```python
from build123d import *

# Parameters (mm, degrees)
SKETCH_1_W      = 45
SKETCH_1_H      = 16
SKETCH_1_R      = 0.5
EXTRUDE_1_DEPTH = 2
EXTRUDE_2_DEPTH = 20
SKETCH_3_W      = 45
SKETCH_3_H      = 16
SKETCH_3_R      = 0.5
EXTRUDE_3_DEPTH = 2


with BuildPart() as part:
    # 草图1 → 凸台-拉伸1 (new body)
    with BuildSketch(Plane.XY):
        Rectangle(SKETCH_1_W, SKETCH_1_H)
        with Locations((-20, -6.5)):
            Circle(SKETCH_1_R, mode=Mode.SUBTRACT)
        with Locations((-20, 6.5)):
            Circle(SKETCH_1_R, mode=Mode.SUBTRACT)
        with Locations((20, 6.5)):
            Circle(SKETCH_1_R, mode=Mode.SUBTRACT)
        with Locations((20, -6.5)):
            Circle(SKETCH_1_R, mode=Mode.SUBTRACT)
    extrude(amount=EXTRUDE_1_DEPTH)

    # 草图2 → 凸台-拉伸2 (add)
    with BuildSketch(Plane.XY.offset(2)):
        Polygon((-18.845299462, 6.5), (-19.422649731, 7.5), (-20.577350269, 7.5), (-21.154700538, 6.5), (-20.577350269, 5.5), (-19.422649731, 5.5), align=None)
        Polygon((19.422649731, 5.5), (18.845299462, 6.5), (19.422649731, 7.5), (20.577350269, 7.5), (21.154700538, 6.5), (20.577350269, 5.5), align=None)
        Polygon((18.845299462, -6.5), (19.422649731, -7.5), (20.577350269, -7.5), (21.154700538, -6.5), (20.577350269, -5.5), (19.422649731, -5.5), align=None)
        Polygon((-19.422649731, -5.5), (-18.845299462, -6.5), (-19.422649731, -7.5), (-20.577350269, -7.5), (-21.154700538, -6.5), (-20.577350269, -5.5), align=None)
    extrude(amount=EXTRUDE_2_DEPTH)

    # 草图3 → 凸台-拉伸3 (add)
    with BuildSketch(Plane.XY.offset(22)):
        Rectangle(SKETCH_3_W, SKETCH_3_H)
        with Locations(Location((20, 6.5, 0), (0, 0, 180))):
            Circle(SKETCH_3_R, mode=Mode.SUBTRACT)
        with Locations(Location((-20, -6.5, 0), (0, 0, 180))):
            Circle(SKETCH_3_R, mode=Mode.SUBTRACT)
        with Locations((-20, 6.5)):
            Circle(SKETCH_3_R, mode=Mode.SUBTRACT)
        with Locations((20, -6.5)):
            Circle(SKETCH_3_R, mode=Mode.SUBTRACT)
    extrude(amount=EXTRUDE_3_DEPTH)


solid = part.part
```
Read the model definition and answer for the solid it produces. Units are mm, in the model's axes. A direction names the side the tool comes from. Give positions to 0.01 mm unless a question says otherwise; leave off trailing zeros. Order: outer loops, then holes, each group sorted by start corner. A loop starts at its lowest first (then second) coordinate and runs counter-clockwise, first axis right, second up. Notation, with made-up numbers: (-39, 27.5) -> (-14, 27.5) arc R21 cw to (-14, 31.5) -> close; hole circle Ø11 at (21, 76). An arc over 180 degrees is marked (long way). Write item = value, one per line.
1. A cutting plane is placed at C-C, the plane x = 5. Write down the section's boundary in (y, z), and give its area (3 significant figures).
Numbers:
outline = (-8, 0) -> (8, 0) -> (8, 2) -> (-8, 2) -> close; (-8, 22) -> (8, 22) -> (8, 24) -> (-8, 24) -> close
area = 64.0 mm²
2. A cutting plane is placed at A-A, the plane y = -1.25. Write down the section's boundary in (x, z), and give its area (3 significant figures).
Numbers:
outline = (-22.5, 0) -> (22.5, 0) -> (22.5, 2) -> (-22.5, 2) -> close; (-22.5, 22) -> (22.5, 22) -> (22.5, 24) -> (-22.5, 24) -> close
area = 180 mm²
3. Straight lines are drawn through the part: line 1 along Y through (x, z) = (20, 1); line 2 along Z through (x, y) = (0, 2.75); line 3 along X through (y, z) = (6.5, 20.5). For each, find the intervals that lie inside material, in ascending order.
Numbers:
line_1 = -8 to -7, -6 to 6, 7 to 8
line_2 = 0 to 2, 22 to 24
line_3 = -21.15 to -18.85, 18.85 to 21.15
4. Given pin 1 (0.5 mm diameter, centred on x = -20, y = -6.5, fed in from -Z); pin 2 (0.9 mm diameter, centred on x = 20.5, z = 10.5, fed in from +Y); pin 3 (8 mm diameter, centred on y = 3, z = 12, fed in from +X), each flat-ended and moving along its own axis, determine where each tip first touches the part or whether it passes through.
Numbers:
pin_1 = 2
pin_2 = 7.5
pin_3 = 21.15
5. A cutting plane is placed at B-B, the plane z = 8. Write down the section's boundary in (x, y).
Numbers:
outline = (-21.15, -6.5) -> (-20.58, -7.5) -> (-19.42, -7.5) -> (-18.85, -6.5) -> (-19.42, -5.5) -> (-20.58, -5.5) -> close; (-21.15, 6.5) -> (-20.58, 5.5) -> (-19.42, 5.5) -> (-18.85, 6.5) -> (-19.42, 7.5) -> (-20.58, 7.5) -> close; (18.85, -6.5) -> (19.42, -7.5) -> (20.58, -7.5) -> (21.15, -6.5) -> (20.58, -5.5) -> (19.42, -5.5) -> close; (18.85, 6.5) -> (19.42, 5.5) -> (20.58, 5.5) -> (21.15, 6.5) -> (20.58, 7.5) -> (19.42, 7.5) -> close
6. The mould has two halves that part along X. Classify faces 1 (the face through (-20.86, -7.01, 11.86)), 2 (the face through (0, 0, 24)), 3 (the face through (-20, -6, 1)), 4 (the face through (20, 6, 1)): +X half, -X half, draft (parallel to the pull), parting line (faces both ways), or undercut.
Numbers:
face_1 = -X half
face_2 = draft
face_3 = undercut
face_4 = undercut
7. For faces 5 (the face through (-20, 7.5, 12)), 6 (the face through (-20.86, 7.01, 11.86)), 7 (the face through (20.86, 7.01, 11.86)), 8 (the face through (20, -6.5, 22)), determine the directions among +Z, -Z, +X, -X, +Y, -Y from which every point of the face is accessible in a straight line to the end or side of a thin tool.
Numbers:
face_5 = +X, -X, +Y
face_6 = -X, +Y
face_7 = +X, +Y
face_8 = +Z
